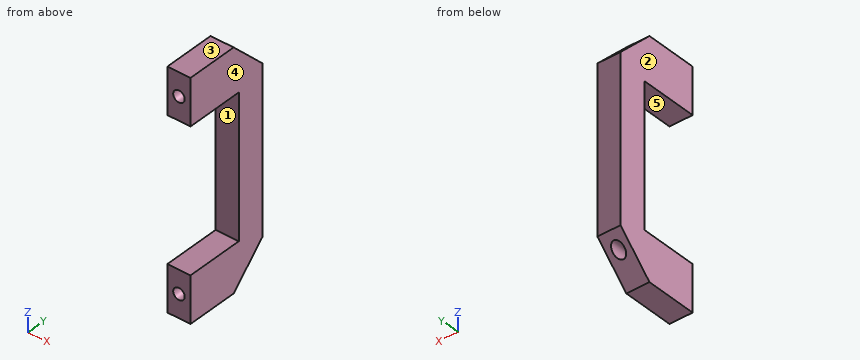
Autodesk Inventor part; units mm, degrees
ref_plane "YZ Plane" through (0, 0, 0) normal (1, 0, 0) x (0, 1, 0)
ref_plane "XZ Plane" through (0, 0, 0) normal (0, 1, 0) x (-1, 0, 0)
ref_plane "XY Plane" through (0, 0, 0) normal (0, 0, 1) x (1, 0, 0)
sketch "Sketch1" plane through (0, 0, 0) normal (0, 0, 1) x (1, 0, 0)
  line L0 (0, 0) -> (-12.7, 0)
  line L1 (-12.7, 0) -> (-12.7, 47.4345)
  line L2 (-12.7, 47.4345) -> (0, 47.4345)
  line L3 (0, 47.4345) -> (0, 0)
  dimension "d0" = 12.7
  dimension "d1" = 47.4345
extrude "Extrusion1" add sketch "Sketch1" along normal blind 128.5875
sketch "Sketch2" plane through (0, 0, 0) normal (1, 0, 0) x (0, 0, -1)
  line L0 (-25.4, 0) -> (-103.1875, 0)
  line L1 (-103.1875, 0) -> (-103.1875, 31.75)
  line L2 (-103.1875, 31.75) -> (-25.4, 31.75)
  line L3 (-25.4, 31.75) -> (-25.4, 0)
  line L4 (0, 47.4345) -> (0, 0)
  line L5 (-128.5875, 0) -> (-128.5875, 47.4345)
  line L6 (0, 0) -> (-128.5875, 0)
  dimension "d4" = 25.4
  dimension "d5" = 25.4
  dimension "d6" = 77.7875
  dimension "d7" = 31.75
  dimension "d8" = 0
extrude "Extrusion2" cut sketch "Sketch2" against normal blind 77.7875
sketch "Sketch3" plane through (-12.7, 47.4345, 0) normal (0, 1, 0) x (1, 0, 0)
  circle A0 centre (6.35, -115.8875) radius 3.175
  circle A1 centre (6.35, -12.7) radius 3.175
  line L0 (0, 0) -> (0, -128.5875)
  line L1 (12.7, -128.5875) -> (0, -128.5875)
  line L2 (0, 0) -> (12.7, 0)
  dimension "d11" = 6.35
  dimension "d12" = 6.35
  dimension "d13" = 6.35
  dimension "d14" = 6.35
  dimension "d15" = 12.7
  dimension "d16" = 12.7
extrude "Extrusion3" cut sketch "Sketch3" against normal blind 77.7875
chamfer "Chamfer1" distance 19.05 angle 45 2 edges at (-6.35, 47.4345, 0) (-6.35, 47.4345, 128.5875)
properties part number "Intake Robustifier"
CAD build for the part. Positions are in the model's coordinates, mm. Face numbers are marked on the shaded views. A direction names the side the tool comes from. Coordinates: 2 decimals unless noted, no trailing zeros. Order: outer loops, then holes, each group sorted by start corner. A loop starts at its lowest first (then second) coordinate and runs counter-clockwise, first axis right, second up. Notation, with made-up numbers: (38, -31.5) -> (85, -31.5) arc R24 ccw to (85, -15.5) -> close; hole circle Ø10 at (12, 11). An arc over 180 degrees is marked (long way). Use one line per item in the form item = value. Start each with the question number.
1) Tool access for the marked faces 4 and 5: list every direction of +Z, -Z, +X, -X, +Y, -Y with a clear straight run to the whole face (end or side of a thin tool).
2) Drill centre lines: L1, parallel to Z at x = -6.35, y = 16 (1 decimal); L2, parallel to Z at x = -1, y = 8.5; L3, parallel to Z at x = -6.35, y = 35 (1 decimal). Where is each one in solid material? Low to high. Write a range as [from, to].
3) Drop flat-ended pins along their axis: pin 1 (2 mm diameter, centred on x = -1.5, z = 16.5, fed in from +Y); pin 2 (5 mm diameter, centred on x = -4.5, z = 80.5, fed in from -Y); pin 3 (1 mm diameter, centred on x = -11, y = 42.5, fed in from -Z); pin 4 (5.5 mm diameter, centred on x = -6.35, z = 115.89, fed in from -Y). Give the stop position or say it passes through.
4) Band-saw the part on C-C on x = -1.25. Give the cut face in (y, z).
5) Band-saw the part on A-A on y = 13.5. State how many separate pieces and enclosed holes the cut face has, then the cut area to 3 significant figures.
6) Band-saw the part on B-B on x = -7.5. Give the cut face in (y, z), then the cut area to 3 significant figures.
7) Pull direction Z, two halves, no side cores. Call the marked faces 1, 2 and 3: +Z half, -Z half, draft (parallel to the pull), parting line (faces both ways), or undercut.
Entries:
q1.face_4 = +Z, -Z, +X, +Y, -Y
q1.face_5 = +X, -X, -Y
q2.L1 = [0, 9.5], [15.9, 25.4], [103.2, 112.7], [119.1, 128.6]
q2.L2 = [0, 25.4], [103.19, 128.59]
q2.L3 = [6.6, 9.5], [15.9, 112.7], [119.1, 122]
q3.pin_1 = 45.88
q3.pin_2 = 31.75
q3.pin_3 = 13.62
q3.pin_4 = through
q4.outline = (0, 0) -> (28.38, 0) -> (47.43, 19.05) -> (47.43, 109.54) -> (28.38, 128.59) -> (0, 128.59) -> (0, 103.19) -> (31.75, 103.19) -> (31.75, 25.4) -> (0, 25.4) -> close
q5.separate_pieces = 2
q5.enclosed_holes = 2
q5.area = 582 mm2
q6.outline = (0, 0) -> (28.38, 0) -> (38.13, 9.74) -> (0, 9.74) -> close; (0, 15.66) -> (44.04, 15.66) -> (47.43, 19.05) -> (47.43, 109.54) -> (44.04, 112.93) -> (0, 112.93) -> (0, 103.19) -> (31.75, 103.19) -> (31.75, 25.4) -> (0, 25.4) -> close; (0, 118.85) -> (38.13, 118.85) -> (28.38, 128.59) -> (0, 128.59) -> close
q6.area = 2,780 mm2
q7.face_1 = undercut
q7.face_2 = draft
q7.face_3 = +Z half
